Could you check a few things on this model? Use its own coordinates, in mm. A direction names the side the tool comes from. Round coordinates to 2 decimals unless told otherwise and drop trailing zeros. Loops run counter-clockwise (first coordinate to the right, second up) from the corner with the lowest first, then second, coordinate; pieces in that order, holes last. Notation, with made-up numbers: (24, 68.5) - (60, 68.5) arc R24 cw to (60, 100.5) - close; hole circle Ø9 at (2, 32.25). An arc over 180 degrees is marked (long way). Use one line per item in the form item = value.
```python
from build123d import *

# Parameters (mm, degrees)
SKETCH1_W           = 57
SKETCH1_H           = 57
BOSS_EXTRUDE1_DEPTH = 57
SKETCH2_R           = 2
CUT_EXTRUDE1_DEPTH  = 70.810457669
CUT_EXTRUDE4_DEPTH  = 53.34
FILLET1_R           = 2.54
SKETCH9_R           = 19.05
BOSS_EXTRUDE2_DEPTH = 1.6
SKETCH10_R          = 3.175
BOSS_EXTRUDE3_DEPTH = 19
CUT_EXTRUDE5_START  = -15
CUT_EXTRUDE5_DEPTH  = 15
CHAMFER1_SIZE       = 0.254
FILLET2_R           = 0.508


with BuildPart() as part:
    # Sketch1 → Boss-Extrude1 (new body)
    with BuildSketch(Plane.XY):
        Rectangle(SKETCH1_W, SKETCH1_H)
    extrude(amount=BOSS_EXTRUDE1_DEPTH)

    # Sketch2 → Cut-Extrude1 (cut, through all)
    with BuildSketch(Plane.XY.offset(57)):
        with Locations((-23.5, 23.5)):
            Circle(SKETCH2_R)
        with Locations((23.5, 23.5)):
            Circle(SKETCH2_R)
        with Locations((23.5, -23.5)):
            Circle(SKETCH2_R)
        with Locations((-23.5, -23.5)):
            Circle(SKETCH2_R)
    extrude(amount=-CUT_EXTRUDE1_DEPTH, mode=Mode.SUBTRACT)

    # Sketch8 → Cut-Extrude4 (cut)
    with BuildSketch(Plane(origin=(0, 0, 0), x_dir=(-1, 0, 0), z_dir=(0, 0, -1))):
        with BuildLine():
            Line((18.5, -28.5), (18.5, -23.5))
            ThreePointArc((18.5, -23.5), (19.964466094, -19.964466094), (23.5, -18.5))
            Line((23.5, -18.5), (28.5, -18.5))
            Line((28.5, -18.5), (28.5, -28.5))
            Line((28.5, -28.5), (18.5, -28.5))
        make_face()
        with BuildLine():
            Line((23.5, 18.5), (28.5, 18.5))
            Line((28.5, 18.5), (28.5, 28.5))
            Line((28.5, 28.5), (18.5, 28.5))
            Line((18.5, 28.5), (18.5, 23.5))
            ThreePointArc((18.5, 23.5), (19.964466094, 19.964466094), (23.5, 18.5))
        make_face()
        with BuildLine():
            Line((-18.5, 23.5), (-18.5, 28.5))
            Line((-18.5, 28.5), (-28.5, 28.5))
            Line((-28.5, 28.5), (-28.5, 18.5))
            Line((-28.5, 18.5), (-23.5, 18.5))
            ThreePointArc((-23.5, 18.5), (-19.964466094, 19.964466094), (-18.5, 23.5))
        make_face()
        with BuildLine():
            Line((-23.5, -18.5), (-28.5, -18.5))
            Line((-28.5, -18.5), (-28.5, -28.5))
            Line((-28.5, -28.5), (-18.5, -28.5))
            Line((-18.5, -28.5), (-18.5, -23.5))
            ThreePointArc((-18.5, -23.5), (-19.964466094, -19.964466094), (-23.5, -18.5))
        make_face()
    extrude(amount=-CUT_EXTRUDE4_DEPTH, mode=Mode.SUBTRACT)

    # Fillet1
    fillet1_edges = [part.edges().sort_by_distance(p)[0] for p in [
        (28.5, -28.5, 55.17),
        (-28.5, -28.5, 55.17),
        (-28.5, 28.5, 55.17),
        (28.5, 28.5, 55.17),
    ]]
    fillet(fillet1_edges, radius=FILLET1_R)

    # Sketch9 → Boss-Extrude2 (add)
    with BuildSketch(Plane.XY.offset(57)):
        with Locations(Location((0, 0, 0), (0, 0, 180))):
            Circle(SKETCH9_R)
    extrude(amount=BOSS_EXTRUDE2_DEPTH)

    # Sketch10 → Boss-Extrude3 (add)
    with BuildSketch(Plane.XY.offset(58.6)):
        Circle(SKETCH10_R)
    extrude(amount=BOSS_EXTRUDE3_DEPTH)

    # Sketch11 → Cut-Extrude5 (cut)
    with BuildSketch(Plane.XY.offset(77.6).offset(CUT_EXTRUDE5_START)):
        with BuildLine():
            Line((1.234908904, -2.925), (1.234908904, 2.925))
            ThreePointArc((1.234908904, 2.925), (3.175, 0), (1.234908904, -2.925))
        make_face()
    extrude(amount=CUT_EXTRUDE5_DEPTH, mode=Mode.SUBTRACT)

    # Chamfer1
    chamfer1_edges = [part.edges().sort_by_distance(p)[0] for p in [
        (19.05, 0, 58.6),
        (-3.175, 0, 77.6),
        (2.645889337, -1.754962853, 62.6),
    ]]
    chamfer(chamfer1_edges, length=CHAMFER1_SIZE)

    # Fillet2
    fillet2_edges = [part.edges().sort_by_distance(p)[0] for p in [
        (0, -28.5, 0),
        (-26, -18.5, 0),
        (-19.964466094, -19.964466094, 0),
        (-18.5, -26, 0),
        (-18.5, -28.5, 26.67),
        (-28.5, -18.5, 26.67),
        (-28.5, 0, 0),
        (0, 28.5, 0),
        (28.5, 0, 0),
        (18.5, -26, 0),
        (19.964466094, -19.964466094, 0),
        (26, -18.5, 0),
        (28.5, -18.5, 26.67),
        (18.5, -28.5, 26.67),
        (26, 18.5, 0),
        (19.964466094, 19.964466094, 0),
        (18.5, 26, 0),
        (18.5, 28.5, 26.67),
        (28.5, 18.5, 26.67),
        (-19.964466094, 19.964466094, 0),
        (-26, 18.5, 0),
        (-18.5, 26, 0),
        (-18.5, 28.5, 26.67),
        (-28.5, 18.5, 26.67),
    ]]
    fillet(fillet2_edges, radius=FILLET2_R)


solid = part.part
```
1. If we section it at A-A, the plane z = 44: Write out the boundary of the cut face in (x, y).
Solution:
outline = (-28.5, -17.99) arc R0.51 ccw to (-27.99, -18.5) - (-23.5, -18.5) arc R5 cw to (-18.5, -23.5) - (-18.5, -27.99) arc R0.51 ccw to (-17.99, -28.5) - (17.99, -28.5) arc R0.51 ccw to (18.5, -27.99) - (18.5, -23.5) arc R5 cw to (23.5, -18.5) - (27.99, -18.5) arc R0.51 ccw to (28.5, -17.99) - (28.5, 17.99) arc R0.51 ccw to (27.99, 18.5) - (23.5, 18.5) arc R5 cw to (18.5, 23.5) - (18.5, 27.99) arc R0.51 ccw to (17.99, 28.5) - (-17.99, 28.5) arc R0.51 ccw to (-18.5, 27.99) - (-18.5, 23.5) arc R5 cw to (-23.5, 18.5) - (-27.99, 18.5) arc R0.51 ccw to (-28.5, 17.99) - close
2. We'd pull the mould along Y, two halves only. Please class faces 1 (the face through (-3.17, 0.14, 65.76)), 2 (the face through (-27.776, -27.736, 55.196)), 3 (the face through (-18.5, -26, 27)), 4 (the face through (-25.498, -23.412, 55.196)): +Y half, -Y half, draft (parallel to the pull), parting line (faces both ways), or undercut.
Solution:
face_1 = parting line
face_2 = -Y half
face_3 = draft
face_4 = undercut
3. On a 3-axis mill with a long thin cutter (end or side, diameter ignored), from which of +Z, -Z, +X, -X, +Y, -Y can I reach the whole of each face in a straight line? I mean faces 5 (the face through (-0.4, 19.4, 57)), 6 (the face through (-26, -18.5, 27)), 7 (the face through (19.93, -20, 26.55)), 8 (the face through (-19.93, 20, 26.55)), 9 (the face through (26, 23, 53.34)). Say none if no direction works.
Solution:
face_5 = +Z
face_6 = -Z, -X, -Y
face_7 = -Z, +X, -Y
face_8 = -Z, -X, +Y
face_9 = -Z, +X, +Y
4. If we section it at C-C, the plane y = 0: Write out the boundary of the cut face in (x, z) (3 decimals).
Solution:
outline = (-28.5, 0.508) arc R0.508 ccw to (-27.992, 0) - (27.992, 0) arc R0.508 ccw to (28.5, 0.508) - (28.5, 57) - (19.05, 57) - (19.05, 58.346) - (18.796, 58.6) - (3.175, 58.6) - (3.175, 62.346) - (2.921, 62.6) - (1.235, 62.6) - (1.235, 77.6) - (-2.921, 77.6) - (-3.175, 77.346) - (-3.175, 58.6) - (-18.796, 58.6) - (-19.05, 58.346) - (-19.05, 57) - (-28.5, 57) - close
5. Please list where these lines run through material, in increasing order: line 1 along Y through (x, z) = (-23.5, 54.7); line 2 along Y through (x, z) = (23, 55).
Solution:
line_1 = -28.5 to -25.5, -21.5 to 21.5, 25.5 to 28.5
line_2 = -28.5 to -25.44, -21.56 to 21.56, 25.44 to 28.5
6. If we section it at D-D, the plane y = -22.5: Count the separate pieces of the cut face and the enclosed holes in it, plus the area to 3 significant figures.
Solution:
separate_pieces = 3
enclosed_holes = 0
area = 2,170 mm^2
7. If we section it at B-B, the plane x = 0: Write out the boundary of the cut face in (y, z) (3 decimals).
Solution:
outline = (-28.5, 0.508) arc R0.508 ccw to (-27.992, 0) - (27.992, 0) arc R0.508 ccw to (28.5, 0.508) - (28.5, 57) - (19.05, 57) - (19.05, 58.346) - (18.796, 58.6) - (3.175, 58.6) - (3.175, 77.346) - (2.921, 77.6) - (-2.921, 77.6) - (-3.175, 77.346) - (-3.175, 58.6) - (-18.796, 58.6) - (-19.05, 58.346) - (-19.05, 57) - (-28.5, 57) - close
8. For P1, Ø12, axis at x = -20.5, y = 12, coming from the +Z side; P2, Ø2, axis at x = -26.5, z = 14, coming from the +Y side; P3, Ø3.5, axis at y = 26, z = 27, coming from the -X side; P4, Ø11.5, axis at x = -23.5, y = -23.5, coming from the -Z side, each with a flat end and sliding along its axis, tell me the tip position at first contact or that it passes through.
Solution:
P1 = 58.6
P2 = 18.5
P3 = -18.5
P4 = 0
